For this review, take the finished solid that the model builds, in its own axes (mm). A direction names the side the tool comes from. Give positions to 0.01 mm unless a question says otherwise; leave off trailing zeros. Order: outer loops, then holes, each group sorted by start corner. A loop starts at its lowest first (then second) coordinate and runs counter-clockwise, first axis right, second up. Notation, with made-up numbers: (56.5, -2.75) - (112.5, -2.75) arc R32 cw to (112.5, 23.25) - close; hole circle Ø4 at (-12.75, 12.25). An arc over 180 degrees is marked (long way). One line per item, written item: value.
```python
from build123d import *

# Parameters (mm, degrees)
BOSS_EXTRUDE1_DEPTH    = 9
M3X0_5_TAPPED_HOLE1_D  = 2.5
M3_CLEARANCE_HOLE2_D   = 3.4
F_25_0MM_DOWEL_HOLE1_D = 25


with BuildPart() as part:
    # Sketch1 → Boss-Extrude1 (new body)
    with BuildSketch(Plane.XY):
        Polygon((0, 0), (45.5, 0), (45.5, 2), (39.5, 2), (39.5, 37), (6, 37), (6, 2), (0, 2), align=None)
    extrude(amount=BOSS_EXTRUDE1_DEPTH)

    # M3x0.5 Tapped Hole1 (through all)
    with Locations(Plane(origin=(36.5, 34, 9), x_dir=(1, 0, 0), z_dir=(0, 0, 1))):
        with Locations((0, 0), (-27.5, -27.5)):
            Hole(M3X0_5_TAPPED_HOLE1_D / 2)

    # M3 Clearance Hole2 (through all)
    with Locations(Plane(origin=(42.5, 2, 4.5), x_dir=(0, 0, 1), z_dir=(0, 1, 0))):
        with Locations((0, 0), (0, -39.5)):
            Hole(M3_CLEARANCE_HOLE2_D / 2)

    # Ø25.0mm Dowel Hole1 (through all)
    with Locations(Plane.XY.offset(9)):
        with Locations((22.75, 20.25)):
            Hole(F_25_0MM_DOWEL_HOLE1_D / 2)


solid = part.part
```
(1) Machinability: for faces 1 (the face through (44, 2, 3)), 2 (the face through (6, 20, 4)), 3 (the face through (9.99, 5.74, 4.44)), which of the approach directions +Z, -Z, +X, -X, +Y, -Y give a long, thin tool a straight path to every point of the face, cutting with its end or side? Answer none if there is none.
Answers below:
face 1: +Z, -Z, +X, +Y
face 2: +Z, -Z, -X, +Y
face 3: +Z, -Z
(2) Wall thickness on line 1 (X direction, y = 20, z = 8.5); line 2 (Y direction, x = 9, z = 8.5); line 3 (Y direction, x = 22.75, z = 6.5): over which ranges is each line inside the solid? List them lowest first. Write a range as from..to.
Answers below:
line 1: x = 6..10.25, 35.25..39.5
line 2: y = 0..5.25, 7.75..37
line 3: y = 0..7.75, 32.75..37
(3) Take a section at A-A (z = 4.5). Write out the cut boundary in (x, y), then the cut area to 3 significant figures.
Answers below:
outline: (0, 0) - (1.3, 0) - (1.3, 2) - (0, 2) - close; (4.7, 0) - (40.8, 0) - (40.8, 2) - (39.5, 2) - (39.5, 37) - (6, 37) - (6, 2) - (4.7, 2) - close; (44.2, 0) - (45.5, 0) - (45.5, 2) - (44.2, 2) - close; hole circle Ø2.5 at (9, 6.5); hole circle Ø25 at (22.75, 20.25); hole circle Ø2.5 at (36.5, 34)
area: 749 mm^2
(4) Take a section at B-B (y = 20.25). Write out the cut boundary in (x, z), then the cut area to 3 significant figures.
Answers below:
outline: (6, 0) - (10.25, 0) - (10.25, 9) - (6, 9) - close; (35.25, 0) - (39.5, 0) - (39.5, 9) - (35.25, 9) - close
area: 76.5 mm^2
(5) Take a section at D-D (z = 1.25). Write out the cut boundary in (x, y), then the cut area to 3 significant figures.
Answers below:
outline: (0, 0) - (45.5, 0) - (45.5, 2) - (39.5, 2) - (39.5, 37) - (6, 37) - (6, 2) - (0, 2) - close; hole circle Ø2.5 at (9, 6.5); hole circle Ø25 at (22.75, 20.25); hole circle Ø2.5 at (36.5, 34)
area: 763 mm^2
(6) For P1, Ø4.5, axis at y = 26, z = 6, coming from the -X side; P2, Ø1.8, axis at x = 4, z = 4, coming from the +Y side; P3, Ø2, axis at x = 9, y = 6.5, coming from the +Z side; P4, Ø2.5, axis at y = 20, z = 5, coming from the +X side, all flat-tipped, find the tip position at first contact; note any pin that passes through.
Answers below:
P1: stops at x = 6
P2: stops at y = 2
P3: passes through
P4: stops at x = 39.5
(7) Draft analysis for pull direction Y (two halves, no side actions). For faces 4 (the face through (32.67, 12.644, 4.437)), 5 (the face through (22, 0, 4)), 6 (the face through (45.5, 1, 4)), state which applies: pulls with the +Y half, pulls with the -Y half, needs draft (parallel to the pull), parting line crosses it, or undercut.
Answers below:
face 4: undercut
face 5: pulls with the -Y half
face 6: needs draft
(8) Take a section at C-C (x = 42.5). Write out the cut boundary in (y, z).
Answers below:
outline: (0, 0) - (2, 0) - (2, 2.8) - (0, 2.8) - close; (0, 6.2) - (2, 6.2) - (2, 9) - (0, 9) - close
